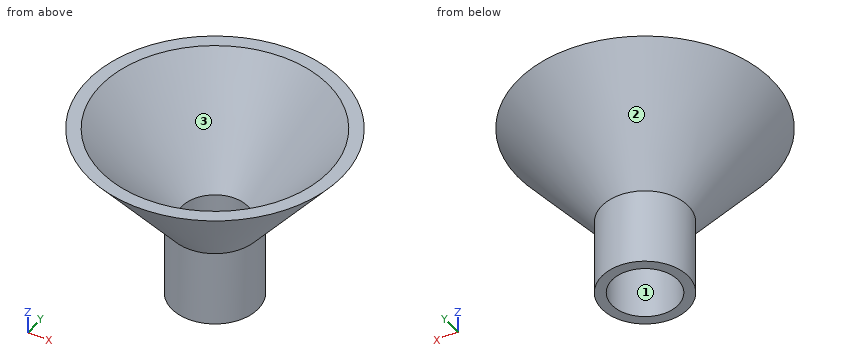
Autodesk Fusion 360 part; units mm, degrees
sketch "Sketch1" plane through (0, 0, 0) normal (0, 0, 1) x (1, 0, 0)
  circle A0 centre (0, 0) radius 8.5
  dimension "d6" = 17
extrude "Extrude1" add sketch "Sketch1" along normal blind 15
ref_plane "WorkPlane1" through (0, 0, 35) normal (0, 0, 1) x (1, 0, 0)
sketch "Sketch2" plane through (0, 0, 35) normal (0, 0, 1) x (1, 0, 0)
  circle A0 centre (0, 0) radius 25
  dimension "d10" = 50
loft "Loft1" add profiles "Sketch2" section 1 section 2 face at (2.7075, 1.6235, 15)
shell "Shell1" thickness 2 removed faces 2 at (2.7075, 1.6235, 0) at (-6.7759, -1.242, 35)
equation "FH = 20 mm"
equation "TL = 15 mm"
equation "WT = 2 mm"
equation "LD = 50 mm"
equation "SD = 17 mm"
equation "d6 = SD"
equation "d7 = TL"
equation "d9 = FH"
equation "d10 = LD"
equation "d11 = WT"
Read the model definition and answer for the solid it produces. Units are mm, in the model's axes. Face numbers are marked on the shaded views. Round coordinates to 2 decimals unless told otherwise and drop trailing zeros. Write each loop counter-clockwise with the first axis right and the second up, starting at its lowest first coordinate (ties: lowest second). Pieces come first, ordered by that corner, then holes. Notation, with made-up numbers: (-27, 65.25) - (-10, 65.25) arc R21 ccw to (-10, 100.25) - close; hole circle Ø8 at (-11, 27.25). An arc over 180 degrees is marked (long way). Use a Markdown table: item, result.
(1) The part is cut by section A-A (x = 0). Write down the section's boundary in (y, z).
Reported:
| item | result |
|---|---|
| outline | (-25, 35) - (-8.5, 15) - (-8.5, 0) - (-6.5, 0) - (-6.5, 15.72) - (-22.41, 35) - close; (6.5, 0) - (8.5, 0) - (8.5, 15) - (25, 35) - (22.41, 35) - (6.5, 15.72) - close |
(2) The mould has two halves that part along Y. Classify the marked faces 1, 2 and 3: released by +Y, released by -Y, zero draft, split by the parting line, or undercut.
Reported:
| item | result |
|---|---|
| face 1 | undercut |
| face 2 | split by the parting line |
| face 3 | undercut |
(3) The part is cut by section C-C (z = 25). Write down the section's boundary in (x, y).
Reported:
| item | result |
|---|---|
| outline | circle Ø33.5 at (0, 0); hole circle Ø28.31 at (0, 0) |
(4) The part is cut by section B-B (z = 7). Write down the section's boundary in (x, y).
Reported:
| item | result |
|---|---|
| outline | circle Ø17 at (0, 0); hole circle Ø13 at (0, 0) |
(5) Each of these flat-tipped pins is pushed along its axis until it touches: pin 1 Ø6 at (y, z) = (11.5, 18.5) entering from +X; pin 2 Ø8 at (x, z) = (-14, 30) entering from -Y; pin 3 Ø1.5 at (x, z) = (-13.5, 22.5) entering from -Y. Where does it stop, or does it pass through?
Reported:
| item | result |
|---|---|
| pin 1 | x = 9.21 |
| pin 2 | y = -20.48 |
| pin 3 | y = -7.78 |
(6) Straight lines are drawn through the part: line 1 along Y through (x, z) = (0, 8); line 2 along X through (y, z) = (-15, 33); line 3 along Y through (x, z) = (2.5, 33). For each, find the intervals that lie inside material, in ascending order. Write a range as [from, to].
Reported:
| item | result |
|---|---|
| line 1 | [-8.5, -6.5], [6.5, 8.5] |
| line 2 | [-17.89, -14.35], [14.35, 17.89] |
| line 3 | [-23.22, -20.61], [20.61, 23.22] |
